Source: CAD feature listing. Evaluate the final solid. Frame: model axes, mm. A direction names the side the tool comes from. Round coordinates to 2 decimals unless told otherwise and drop trailing zeros. Order: outer loops, then holes, each group sorted by start corner. A loop starts at its lowest first (then second) coordinate and runs counter-clockwise, first axis right, second up. Notation, with made-up numbers: (12, 1) - (49, 1) arc R14 ccw to (49, 17) - close; hole circle Ø1 at (18, 25.5). An arc over 180 degrees is marked (long way). Return JSON: item names as keys, results as strings. Group by question number.
1) Ray query, line 1 (Y direction, x = -25.5, z = 27.5); line 2 (Y direction, x = 19, z = 33); line 3 (X direction, y = -45, z = 33). Return the intervals inside material, ascending. Write a range as from..to.
2) Access query for faces 1 (the cylindrical face through (-12.15, -76.07, 4.54)), 2 (the flat face through (-44.43, -23.34, 21.79)), 3 (the flat face through (2, -45, 50.8)), 4 (the flat face through (25.327, -34, 18)), 5 (the flat face through (21.61, 19.78, 19.14)). Directions: +Z, -Z, +X, -X, +Y, -Y. A direction counts if a zero-diameter tool reaches every point of the face in a straight line with its end or side. Return the directions, or none.
3) Section D-D, the plane z = 20.5. Return loops of the section in (x, y), plus the area to 3 significant figures.
4) Contact query for flat-ended pins moving along their axis: P1, Ø2, axis at y = -48.5, z = 45, coming from the +X side; P2, Ø1, axis at y = 27, z = 7, coming from the +X side; P3, Ø8, axis at x = 5.5, z = 14, coming from the -Y side; P4, Ø6, axis at x = -19.5, y = -12, coming from the -Z side. Output: stop coordinate, or through.
5) Section A-A, the plane z = 45. Return loops of the section in (x, y), plus the area to 3 significant figures.
```python
from build123d import *

# Parameters (mm, degrees)
F0_W        = 88.9000063658
F0_H        = 152.4
F1_DEPTH    = 6.35
F2_DEPTH    = 25.4
F3_DEPTH    = 50.8
F4_R        = 6.34999
F5_C1_SIZE2 = 12.7
F5_C1_SIZE  = 7.3323484187
F5_C2_SIZE2 = 7.3323484187
F5_C2_SIZE  = 12.7
F5_C3_SIZE2 = 7.3323484187
F5_C3_SIZE  = 12.7
F5_C4_SIZE2 = 7.3323484187
F5_C4_SIZE  = 12.7
F5_C5_SIZE2 = 12.7
F5_C5_SIZE  = 7.3323484187
F5_C6_SIZE2 = 7.3323484187
F5_C6_SIZE  = 12.7
F6_SIZE2    = 7.3323484187
F6_SIZE     = 12.7


# Not quite as in the source:
# - a fillet or chamfer is up to 0.001 mm smaller than in the source, because OpenCascade refuses the exact size


with BuildPart() as f1:
    # F0 (on Top) → F1 (new body)
    with BuildSketch(Plane.XY):
        with Locations((-12.7734099567, -1.7824335903)):
            Rectangle(F0_W, F0_H)
        Polygon((-50.8734099567, 23.6175632268), (-50.8734099567, 68.0675632268), (-12.7734099567, 68.0675632268), (25.3265900433, 68.0675632268), (25.3265900433, -27.1824304074), (25.3265900433, -71.6324304074), (-12.7734099567, -71.6324304074), (-50.8734099567, -71.6324304074), align=None, mode=Mode.SUBTRACT)
    extrude(amount=F1_DEPTH)

    # F0 (on Top) → F2 (join)
    with BuildSketch(Plane.XY):
        with BuildLine():
            Line((25.3265900433, 68.0675632268), (-12.7734099567, 68.0675632268))
            Line((-12.7734099567, 68.0675632268), (-12.7734099567, 36.3175632268))
            ThreePointArc((-12.7734099567, 36.3175632268), (-16.4931538356, 27.3373071057), (-25.4734099567, 23.6175632268))
            Line((-25.4734099567, 23.6175632268), (-50.8734099567, 23.6175632268))
            Line((-50.8734099567, 23.6175632268), (-50.8734099567, -71.6324304074))
            Line((-50.8734099567, -71.6324304074), (-12.7734099567, -71.6324304074))
            Line((-12.7734099567, -71.6324304074), (-12.7734099567, -39.8824304074))
            ThreePointArc((-12.7734099567, -39.8824304074), (-9.0536660778, -30.9021742863), (-0.0734099567, -27.1824304074))
            Line((-0.0734099567, -27.1824304074), (25.3265900433, -27.1824304074))
            Line((25.3265900433, -27.1824304074), (25.3265900433, 68.0675632268))
        make_face()
    extrude(amount=F2_DEPTH)

    # F0 (on Top) → F3 (join)
    with BuildSketch(Plane.XY):
        with BuildLine():
            Line((-12.7734099567, 68.0675632268), (-50.8734099567, 68.0675632268))
            Line((-50.8734099567, 68.0675632268), (-50.8734099567, 23.6175632268))
            Line((-50.8734099567, 23.6175632268), (-25.4734099567, 23.6175632268))
            ThreePointArc((-25.4734099567, 23.6175632268), (-16.4931538356, 27.3373071057), (-12.7734099567, 36.3175632268))
            Line((-12.7734099567, 36.3175632268), (-12.7734099567, 68.0675632268))
        make_face()
        with BuildLine():
            Line((25.3265900433, -71.6324304074), (25.3265900433, -27.1824304074))
            Line((25.3265900433, -27.1824304074), (-0.0734099567, -27.1824304074))
            ThreePointArc((-0.0734099567, -27.1824304074), (-9.0536660778, -30.9021742863), (-12.7734099567, -39.8824304074))
            Line((-12.7734099567, -39.8824304074), (-12.7734099567, -71.6324304074))
            Line((-12.7734099567, -71.6324304074), (25.3265900433, -71.6324304074))
        make_face()
    extrude(amount=F3_DEPTH)

    # F4 (radius 6.35 in the source; OpenCascade refuses exactly that, so slightly less here)
    f4_edges = [f1.edges().sort_by_distance(p)[0] for p in [
        (31.676593, -1.782434, 6.35),
        (-12.77341, -77.982434, 6.35),
        (-57.223413, -1.782434, 6.35),
        (-12.77341, 74.417566, 6.35),
    ]]
    fillet(f4_edges, radius=F4_R)

    # F5: chamfer of 12.7 x 7.3323484187 on 6 edges, made by hand

    # F5_c1
    f5_c1_edges = [f1.edges().sort_by_distance(p)[0] for p in [
        (-50.8734099567, -24.0074335903, 25.4),
    ]]
    f5_c1_side = f1.faces().sort_by_distance((-50.8734099567, -24.0074335903, 25.2533530316))[0]
    chamfer(f5_c1_edges, length=F5_C1_SIZE, length2=F5_C1_SIZE2, reference=f5_c1_side)

    # F5_c2
    f5_c2_edges = [f1.edges().sort_by_distance(p)[0] for p in [
        (-31.8234099567, 68.0675632268, 50.8),
    ]]
    f5_c2_side = f1.faces().sort_by_distance((-31.8234099567, 68.0675632268, 50.6533530316))[0]
    chamfer(f5_c2_edges, length=F5_C2_SIZE, length2=F5_C2_SIZE2, reference=f5_c2_side)

    # F5_c3
    f5_c3_edges = [f1.edges().sort_by_distance(p)[0] for p in [
        (25.3265900433, -49.4074304074, 50.8),
    ]]
    f5_c3_side = f1.faces().sort_by_distance((25.3265900433, -49.4074304074, 50.6533530316))[0]
    chamfer(f5_c3_edges, length=F5_C3_SIZE, length2=F5_C3_SIZE2, reference=f5_c3_side)

    # F5_c4
    f5_c4_edges = [f1.edges().sort_by_distance(p)[0] for p in [
        (25.3265900433, 20.4425664097, 25.4),
    ]]
    f5_c4_side = f1.faces().sort_by_distance((25.3265900433, 20.4425664097, 25.2533530316))[0]
    chamfer(f5_c4_edges, length=F5_C4_SIZE, length2=F5_C4_SIZE2, reference=f5_c4_side)

    # F5_c5
    f5_c5_edges = [f1.edges().sort_by_distance(p)[0] for p in [
        (-25.4734099567, -71.6324304074, 25.4),
    ]]
    f5_c5_side = f1.faces().sort_by_distance((-25.4734099567, -71.6324304074, 25.2533530316))[0]
    chamfer(f5_c5_edges, length=F5_C5_SIZE, length2=F5_C5_SIZE2, reference=f5_c5_side)

    # F5_c6
    f5_c6_edges = [f1.edges().sort_by_distance(p)[0] for p in [
        (2.610415834, -71.6324304074, 50.8),
    ]]
    f5_c6_side = f1.faces().sort_by_distance((2.610415834, -71.6324304074, 50.6533530316))[0]
    chamfer(f5_c6_edges, length=F5_C6_SIZE, length2=F5_C6_SIZE2, reference=f5_c6_side)

    # F6
    f6_edges = [f1.edges().sort_by_distance(p)[0] for p in [
        (-50.87341, 42.176389, 50.8),
    ]]
    f6_side = f1.faces().sort_by_distance((-50.87341, 66.601552, 22.225))[0]
    chamfer(f6_edges, length=F6_SIZE, length2=F6_SIZE2, reference=f6_side)


solid = f1.part
```
Geometry check:
{
 "1": {"line 1": "23.62..68.07", "line 2": "-71.63..-27.18", "line 3": "-12.77..25.33"},
 "2": {"face 1": "+Z, +X, -X, -Y", "face 2": "+Z, -X, -Y", "face 3": "+Z, +X, -X, +Y, -Y", "face 4": "+Z, +X, +Y, -Y", "face 5": "+Z, +X, +Y"},
 "3": {"outline": "(-50.87, 23.62) - (-46.66, 23.62) - (-46.66, -67.42) - (-12.77, -67.42) - (-12.77, -71.63) - (25.33, -71.63) - (25.33, -27.18) - (20.82, -27.18) - (20.82, 68.07) - (-50.87, 68.07) - close", "area": "9,670 mm2"},
 "4": {"P1": "x = 21.92", "P2": "x = 25.33", "P3": "y = -71.63", "P4": "z = 0"},
 "5": {"outline": "(-46.89, 23.62) - (-25.47, 23.62) arc R12.7 ccw to (-12.77, 36.32) - (-12.77, 64.08) - (-46.89, 64.08) - close; (-12.77, -67.65) - (21.34, -67.65) - (21.34, -27.18) - (-0.07, -27.18) arc R12.7 ccw to (-12.77, -39.88) - close", "area": "2,690 mm2"}
}
